```python
from build123d import *

# Parameters (mm, degrees)
CUT_EXTRUDE1_DEPTH = 17.5


with BuildPart() as part:
    # Sketch1 → Revolve1 (revolve)
    with BuildSketch(Plane.XY, mode=Mode.PRIVATE) as revolve1_sk:
        Polygon((0, 0), (0, 5), (50, 5), (52, 3), (60.162162162, 3), (60.162162162, 0), align=None)
    revolve(revolve1_sk.sketch.rotate(Axis((60.162162162, 0, 0), (-1, 0, 0)), 90), axis=Axis((60.162162162, 0, 0), (-1, 0, 0)))

    # Sketch2 → Cut-Extrude1 (cut, symmetric)
    with BuildSketch(Plane.XY):
        Polygon((6.5, -5), (10.64, -0.86), (39.36, -0.86), (43.5, -5), align=None)
    extrude(amount=CUT_EXTRUDE1_DEPTH, both=True, mode=Mode.SUBTRACT)


solid = part.part
```
Build history of the part. All positions in model axes, mm. A direction names the side the tool comes from. Give positions to 0.01 mm unless a question says otherwise; leave off trailing zeros. Loops run counter-clockwise (first coordinate to the right, second up) from the corner with the lowest first, then second, coordinate; pieces in that order, holes last.
Item 1: Slice it at A-A, the plane z = 0. List the corners of the cut face in (x, y).
Answers follow:
outline: (0, -5) - (6.5, -5) - (10.64, -0.86) - (39.36, -0.86) - (43.5, -5) - (50, -5) - (52, -3) - (60.16, -3) - (60.16, 3) - (52, 3) - (50, 5) - (0, 5) - close
Item 2: Flat gauge pins, fed straight in: pin 1 (3 mm diameter, centred on x = 21, z = -1, fed in from -Y); pin 2 (4 mm diameter, centred on x = 51, y = 3, fed in from -Z). Where does each tip first touch, or does it go through?
Answers follow:
pin 1: stops at y = -0.86
pin 2: stops at z = -4.84
Item 3: Which spindle directions (+Z, -Z, +X, -X, +Y, -Y) get a long thin tool onto all of the face, cutting with end or side? Do faces 4 (the face through (25.35, 4.88, 1.08)), 5 (the face through (9, -2.5, 0.1)). Say none if no direction does.
Answers follow:
face 4: +X, -X
face 5: +Z, -Z, -Y
Item 4: Slice it at C-C, the plane x = 34. List the corners of the cut face in (y, z), and give its area (3 significant figures).
Answers follow:
outline: (-0.86, -4.93) arc R5 ccw (long way) to (-0.86, 4.93) - close
area: 47.8 mm2
Item 5: Slice it at B-B, the plane y = 0. List the corners of the cut face in (x, z), and give its area (3 significant figures).
Answers follow:
outline: (0, -5) - (50, -5) - (52, -3) - (60.16, -3) - (60.16, 3) - (52, 3) - (50, 5) - (0, 5) - close
area: 565 mm2
Item 6: Slice it at D-D, the plane x = 54.5. List the corners of the cut face in (y, z), and give its area (3 significant figures).
Answers follow:
outline: circle Ø6 at (0, 0)
area: 28.3 mm2
Item 7: Drill centre lines: line 1 (Z direction, x = 9, y = -0.25); line 2 (X direction, y = -4.5, z = 1.75); line 3 (Y direction, x = 31, z = -4). Where is each one in solid material? Low to high.
Answers follow:
line 1: z = -4.99 to 4.99
line 2: x = 0 to 7, 43 to 50.17
line 3: y = -0.86 to 3
Item 8: Pull direction X, two halves, no side cores. Call faces 1 (the face through (60.162, 0, 0)), 2 (the face through (56.14, -0.9, -2.86)), 3 (the face through (25, -0.86, 0)): released by +X, released by -X, zero draft, split by the parting line, or undercut.
Answers follow:
face 1: released by +X
face 2: zero draft
face 3: undercut
